For this review, take the finished solid that the model builds, in its own axes (mm). A direction names the side the tool comes from. Coordinates: 2 decimals unless noted, no trailing zeros. Loops run counter-clockwise (first coordinate to the right, second up) from the corner with the lowest first, then second, coordinate; pieces in that order, holes last. Notation, with made-up numbers: M 35,11.5 L 41,11.5 A30 ccw 41,46.5 Z; hole C 64.5,33 d1. An arc over 180 degrees is marked long. Put each result on its own line as item: value.
```python
from build123d import *

# Parameters (mm, degrees)
F0_R     = 35
F0_W     = 2
F0_H     = 3
F1_DEPTH = 18
F2_R     = 35
F2_R_2   = 30.5
F3_DEPTH = 31
F5_DEPTH = 5.7


with BuildPart() as f1:
    # F0 (on Top) → F1 (new body)
    with BuildSketch(Plane.XY):
        Circle(F0_R)
        with BuildLine():
            ThreePointArc((-5, 30.0873727667), (0, 30.5), (5, 30.0873727667))
            Line((5, 30.0873727667), (9, 30.0873727667))
            Line((9, 30.0873727667), (9, 29.1418942418))
            ThreePointArc((9, 29.1418942418), (24.5433290325, 18.1073189622), (30.5, 0))
            ThreePointArc((30.5, 0), (24.5433290325, -18.1073189622), (9, -29.1418942418))
            ThreePointArc((9, -29.1418942418), (7.0159448694, -29.6820908561), (5, -30.0873727667))
            ThreePointArc((5, -30.0873727667), (0, -30.5), (-5, -30.0873727667))
            Line((-5, -30.0873727667), (-9, -30.0876272333))
            Line((-9, -30.0876272333), (-9, -29.1418942418))
            ThreePointArc((-9, -29.1418942418), (-30.5, 0), (-9, 29.1418942418))
            Line((-9, 29.1418942418), (-9, 30.0873727667))
            Line((-9, 30.0873727667), (-5, 30.0873727667))
        make_face(mode=Mode.SUBTRACT)
        with BuildLine():
            Line((-5, 30.0873727667), (5, 30.0873727667))
            ThreePointArc((5, 30.0873727667), (0, 30.5), (-5, 30.0873727667))
        make_face()
        with BuildLine():
            Line((9, 30.0873727667), (5, 30.0873727667))
            ThreePointArc((5, 30.0873727667), (7.0159448694, 29.6820908561), (9, 29.1418942418))
            Line((9, 29.1418942418), (9, 30.0873727667))
        make_face()
        with BuildLine():
            ThreePointArc((9, 29.1418942418), (7.0159448694, 29.6820908561), (5, 30.0873727667))
            Line((5, 30.0873727667), (5, 21.0873727667))
            Line((5, 21.0873727667), (5, 15.0873727667))
            Line((5, 15.0873727667), (5, -6.0873727667))
            Line((5, -6.0873727667), (5, -9.0873727667))
            Line((5, -9.0873727667), (5, -14.0873727667))
            Line((5, -14.0873727667), (5, -30.0873727667))
            ThreePointArc((5, -30.0873727667), (7.0159448694, -29.6820908561), (9, -29.1418942418))
            Line((9, -29.1418942418), (9, 29.1418942418))
        make_face()
        with BuildLine():
            Line((-5, 21.0873727667), (-5, 30.0873727667))
            ThreePointArc((-5, 30.0873727667), (-7.0159448694, 29.6820908561), (-9, 29.1418942418))
            Line((-9, 29.1418942418), (-9, -29.1418942418))
            ThreePointArc((-9, -29.1418942418), (-7.0159448694, -29.6820908561), (-5, -30.0873727667))
            Line((-5, -30.0873727667), (-5, -14.0873727667))
            Line((-5, -14.0873727667), (-5, -9.0873727667))
            Line((-5, -9.0873727667), (-5, -6.0873727667))
            Line((-5, -6.0873727667), (-5, 15.0873727667))
            Line((-5, 15.0873727667), (-5, 21.0873727667))
        make_face()
        with BuildLine():
            ThreePointArc((-9, 29.1418942418), (-7.0159448694, 29.6820908561), (-5, 30.0873727667))
            Line((-5, 30.0873727667), (-9, 30.0873727667))
            Line((-9, 30.0873727667), (-9, 29.1418942418))
        make_face()
        Polygon((5, 15.0873727667), (5, 21.0873727667), (0, 21.0873727667), (-5, 21.0873727667), (-5, 15.0873727667), (0, 15.0873727667), align=None)
        with BuildLine():
            ThreePointArc((-5, -30.0873727667), (-7.0159448694, -29.6820908561), (-9, -29.1418942418))
            Line((-9, -29.1418942418), (-9, -30.0876272333))
            Line((-9, -30.0876272333), (-5, -30.0873727667))
        make_face()
        with BuildLine():
            ThreePointArc((-5, -30.0873727667), (0, -30.5), (5, -30.0873727667))
            Line((5, -30.0873727667), (-5, -30.0873727667))
        make_face()
        with Locations((4, -7.5873727667)):
            Rectangle(F0_W, F0_H)
        with Locations((-4, -7.5873727667)):
            Rectangle(F0_W, F0_H)
        Polygon((0, -14.0873727667), (5, -14.0873727667), (5, -9.0873727667), (3, -9.0873727667), (0, -9.0873727667), (-3, -9.0873727667), (-5, -9.0873727667), (-5, -14.0873727667), align=None)
    extrude(amount=F1_DEPTH)

    # F2 (on Top) → F3 (join)
    with BuildSketch(Plane.XY):
        Circle(F2_R)
        Circle(F2_R_2, mode=Mode.SUBTRACT)
    extrude(amount=F3_DEPTH)

    # F4 (on Top) → F5 (join)
    with BuildSketch(Plane.XY):
        with BuildLine():
            ThreePointArc((-14.2633631023, 31.9617970867), (0, 35), (14.2633631023, 31.9617970867))
            Line((14.2633631023, 31.9617970867), (0, 56.6666666667))
            Line((0, 56.6666666667), (-14.2633631023, 31.9617970867))
        make_face()
    extrude(amount=F5_DEPTH)


solid = f1.part
```
(1) Add section B-B (z = 21). Write out the cut boundary in (x, y).
Determined:
outline: C 0,0 d70; hole C 0,0 d61
(2) Add section A-A (z = 15). Write out the cut boundary in (x, y).
Determined:
outline: C 0,0 d70; hole M -9,-29.14 L -9,29.14 A30.5 ccw Z; hole M -5,-30.09 L 5,-30.09 L 5,-14.09 L -5,-14.09 Z; hole M -5,-6.09 L -3,-6.09 L -3,-9.09 L 3,-9.09 L 3,-6.09 L 5,-6.09 L 5,15.09 L -5,15.09 Z; hole M -5,21.09 L 5,21.09 L 5,30.09 L -5,30.09 Z; hole M 9,-29.14 A30.5 ccw 9,29.14 Z
(3) Wall thickness on line 1 along Y through (x, z) = (0, 10.5); line 2 along X through (y, z) = (6, 16.5); line 3 along X through (y, z) = (0, 22): over which ranges is each line inside the solid? List them lowest first. Write a range as [from, to].
Determined:
line 1: y = [-35, -30.09], [-14.09, -9.09], [15.09, 21.09], [30.09, 35]
line 2: x = [-34.48, -29.9], [-9, -5], [5, 9], [29.9, 34.48]
line 3: x = [-35, -30.5], [30.5, 35]
(4) Add section D-D (z = 2). Write out the cut boundary in (x, y), plus the area to 3 significant figures.
Determined:
outline: M -14.26,31.96 A35 ccw long 14.26,31.96 L 0,56.67 Z; hole M -9,-29.14 L -9,29.14 A30.5 ccw Z; hole M -5,-30.09 L 5,-30.09 L 5,-14.09 L -5,-14.09 Z; hole M -5,-6.09 L -3,-6.09 L -3,-9.09 L 3,-9.09 L 3,-6.09 L 5,-6.09 L 5,15.09 L -5,15.09 Z; hole M -5,21.09 L 5,21.09 L 5,30.09 L -5,30.09 Z; hole M 9,-29.14 A30.5 ccw 9,29.14 Z
area: 1,820 mm^2
(5) Tool access review of faces 5 (the flat face through (3, -8, 9)), 6 (the flat face through (-11, 29, 31)), 7 (the flat face through (-6, 0, 18)): name each direction out of +Z, -Z, +X, -X, +Y, -Y from which nothing blocks a thin tool from reaching the whole face with its end or side.
Determined:
face 5: +Z, -Z
face 6: +Z, +X, -X, +Y, -Y
face 7: +Z
(6) Add section C-C (y = 34). Write out the cut boundary in (x, z).
Determined:
outline: M -13.09,0 L 13.09,0 L 13.09,5.7 L 8.31,5.7 L 8.31,31 L -8.31,31 L -8.31,5.7 L -13.09,5.7 Z
(7) For pin 1 (12 mm diameter, centred on x = 19, z = 18, fed in from -Y); pin 2 (2 mm diameter, centred on x = -4, z = 9.5, fed in from +Y); pin 3 (1 mm diameter, centred on x = -2.5, z = 15.5, fed in from -Y), all flat-tipped, find the tip position at first contact; note any pin that passes through.
Determined:
pin 1: stops at y = -32.5
pin 2: stops at y = 34.87
pin 3: stops at y = -34.94
(8) Draft analysis for pull direction X (two halves, no side actions). For faces 1 (the flat face through (7.23, 44.14, 2.81)), 2 (the flat face through (-8, 11, 0)), 3 (the flat face through (0, -14.087, 9)), 4 (the cylindrical face through (-7.587, -34.168, 15.283)), state which applies: +X half, -X half, draft (parallel to the pull), parting line (faces both ways), or undercut.
Determined:
face 1: +X half
face 2: draft
face 3: undercut
face 4: parting line
